Autodesk Fusion 360 part; units mm, degrees
sketch "Sketch1" plane through (0, 0, 0) normal (0, 0, 1) x (1, 0, 0)
  circle A0 centre (0, 0) radius 1.5
  dimension "d1" = 3
extrude "Extrude1" add sketch "Sketch1" along normal blind 19 makes body 1
sketch "Sketch2" plane through (0, 0, 19) normal (0, 0, 1) x (-1, 0, 0)
  circle A0 centre (0, 0) radius 1.5
  circle A1 centre (0, 0) radius 2.5
  dimension "d4" = 5
extrude "Extrude2" add sketch "Sketch2" along normal blind 1 separate body makes body 2
extrude "Extrude3" add 1 faces at (0.567, -0.5383, 19) along direction (0, 0, 1) blind 1 on bodies 1 bodies 1 2
thread "Thread1"
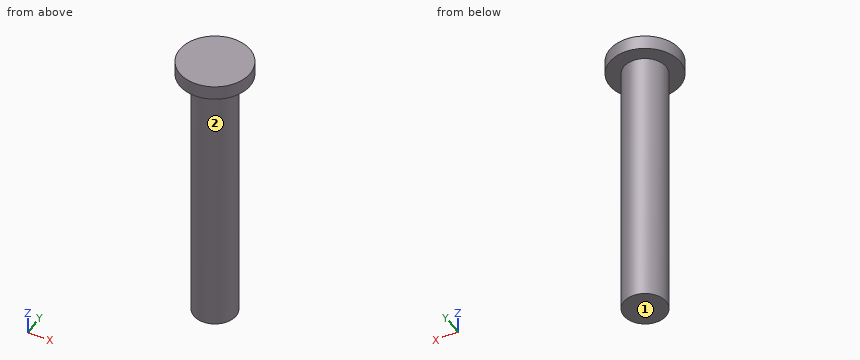
The model under review builds one solid part; all positions refer to its coordinate system, in mm. Face numbers are marked on the shaded views. A direction names the side the tool comes from. Round coordinates to 2 decimals unless told otherwise and drop trailing zeros. Write each loop counter-clockwise with the first axis right and the second up, starting at its lowest first coordinate (ties: lowest second). Pieces come first, ordered by that corner, then holes. Notation, with made-up numbers: (9.5, 38) -> (60.5, 38) arc R12 ccw to (60.5, 46) -> close; hole circle Ø7 at (21.25, 84). An arc over 180 degrees is marked (long way). Use CSV: the item, a comma, the result in double quotes.
Q1. Consider section C-C (z = 11.25). Give the boundary of the cut face in (x, y).
Checks:
outline,"circle Ø3 at (0, 0)"
Q2. To check wall thickness, follow probe 1 along Z at (x, y) = (2.1, -0.25); probe 2 along X at (y, z) = (-0.35, 5.5); probe 3 along Y at (x, z) = (1.3, 6.75). State the ranges of each line that lie inside material, in increasing order. Write a range as [from, to].
Checks:
probe 1,"[19, 20]"
probe 2,"[-1.46, 1.46]"
probe 3,"[-0.75, 0.75]"
Q3. For the marked faces 1 and 2, list the 3-axis set-ups (+Z, -Z, +X, -X, +Y, -Y) from which the entire face can be reached by the end or side of a thin tool; tool diameter is ignored.
Checks:
face 1,"-Z, +X, -X, +Y, -Y"
face 2,"-Z"
Q4. Consider section A-A (y = 0). Give the boundary of the cut face in (x, z).
Checks:
outline,"(-2.5, 19) -> (-1.5, 19) -> (-1.5, 0) -> (1.5, 0) -> (1.5, 19) -> (2.5, 19) -> (2.5, 20) -> (-2.5, 20) -> close"
Q5. For pin 1 Ø1.5 at (x, y) = (-1.5, -0.5) entering from -Z; pin 2 Ø1 at (x, z) = (-1, 12) entering from +Y, all flat-tipped, find the tip position at first contact; note any pin that passes through.
Checks:
pin 1,"z = 0"
pin 2,"y = 1.41"
